Job drawing, mm, ordinate dimensions from the low corner. One solid piece. A direction names the side the tool comes from. Round coordinates to 2 decimals unless told otherwise and drop trailing zeros. Loops run counter-clockwise (first coordinate to the right, second up) from the corner with the lowest first, then second, coordinate; pieces in that order, holes last.
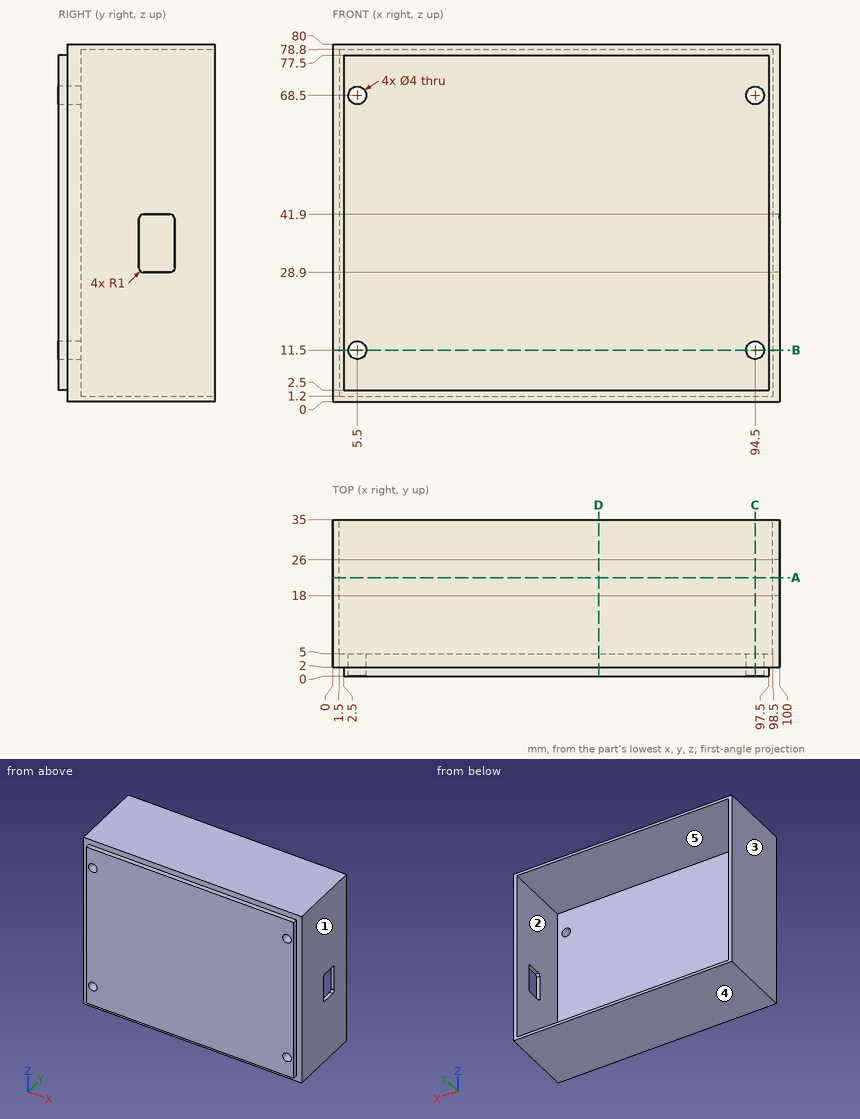
1) Slice it at C-C, the plane x = 94.5. Give the cut face in (y, z).
Values:
outline: (0, 2.5) - (2, 2.5) - (2, 0) - (35, 0) - (35, 1.2) - (5, 1.2) - (5, 9.5) - (0, 9.5) - close; (0, 13.5) - (5, 13.5) - (5, 66.5) - (0, 66.5) - close; (0, 70.5) - (5, 70.5) - (5, 78.8) - (35, 78.8) - (35, 80) - (2, 80) - (2, 77.5) - (0, 77.5) - close
2) Tool access for the marked faces 1 and 2: list every direction of +Z, -Z, +X, -X, +Y, -Y with a clear straight run to the whole face (end or side of a thin tool).
Values:
face 1: +Z, -Z, +X, +Y, -Y
face 2: +Y
3) Wall check: line 1 along X through (y, z) = (3.8, 68.5); line 2 along Z through (x, y) = (29.5, 23.5); line 3 along X through (y, z) = (6, 9). Give the ranges that are in metal, low to high.
Values:
line 1: x = 0 to 3.5, 7.5 to 92.5, 96.5 to 100
line 2: z = 0 to 1.2, 78.8 to 80
line 3: x = 0 to 1.5, 98.5 to 100
4) Slice it at D-D, the plane x = 59.5. Give the cut face in (y, z).
Values:
outline: (0, 2.5) - (2, 2.5) - (2, 0) - (35, 0) - (35, 1.2) - (5, 1.2) - (5, 78.8) - (35, 78.8) - (35, 80) - (2, 80) - (2, 77.5) - (0, 77.5) - close
5) Drop flat-ended pins along their axis: pin 1 Ø10 at (x, z) = (20, 65) entering from +Y; pin 2 Ø1.6 at (x, y) = (67, 1) entering from +Z; pin 3 Ø0.6 at (y, z) = (1, 32) entering from +X. Give the stop position or say it passes through.
Values:
pin 1: stops at y = 5
pin 2: stops at z = 77.5
pin 3: stops at x = 97.5
6) Slice it at B-B, the plane z = 11.5. Give the cut face in (x, y), then the cut area to 3 significant figures.
Values:
outline: (0, 2) - (2.5, 2) - (2.5, 0) - (3.5, 0) - (3.5, 5) - (1.5, 5) - (1.5, 35) - (0, 35) - close; (7.5, 0) - (92.5, 0) - (92.5, 5) - (7.5, 5) - close; (96.5, 0) - (97.5, 0) - (97.5, 2) - (100, 2) - (100, 35) - (98.5, 35) - (98.5, 5) - (96.5, 5) - close
area: 540 mm2
7) Slice it at A-A, the plane y = 22. Give the cut face in (x, z), then the cut area to 3 significant figures.
Values:
outline: (0, 0) - (100, 0) - (100, 28.9) - (98.5, 28.9) - (98.5, 1.2) - (1.5, 1.2) - (1.5, 78.8) - (98.5, 78.8) - (98.5, 41.9) - (100, 41.9) - (100, 80) - (0, 80) - close
area: 453 mm2
8) Mould opens along X. For the marked faces 3, 4 and 5 say: released by +X, released by -X, zero draft, split by the parting line, or undercut.
Values:
face 3: released by -X
face 4: zero draft
face 5: undercut
